Autodesk Inventor part; units mm, degrees
ref_plane "YZ Plane" through (0, 0, 0) normal (1, 0, 0) x (0, 1, 0)
ref_plane "XZ Plane" through (0, 0, 0) normal (0, 1, 0) x (-1, 0, 0)
ref_plane "XY Plane" through (0, 0, 0) normal (0, 0, 1) x (1, 0, 0)
sketch "Sketch1" plane through (0, 0, 0) normal (0, 1, 0) x (-1, 0, 0)
  circle A0 centre (0, 0) radius 2.0828
  dimension "d4" = 4.1656
extrude "Body" add sketch "Sketch1" along normal blind 6.35
sketch "Sketch2" plane through (0, 0, 0) normal (1, 0, 0) x (0, 1, 0)
  line L0 (6.35, -2.0828) -> (6.35, 2.0828)
  line L1 (6.35, 0) -> (6.35, -3.9624)
  line L2 (6.35, -3.9624) -> (6.731, -3.9624)
  arc A0 (6.731, -3.9624) -> (8.5598, -2.0828) centre (4.5388, 0) ccw
  line L3 (8.5598, -2.0828) -> (8.5598, -1.1938)
  line L4 (8.5598, -1.1938) -> (7.4676, -1.1938)
  line L5 (7.4676, -1.1938) -> (7.0866, -0.5588)
  line L6 (7.0866, -0.5588) -> (7.0866, 0)
  line L7 (7.0866, 0) -> (6.35, 0)
  point P0 (0, 0)
  dimension "d5" = 3.9624
  dimension "d6" = 0.381
  dimension "d13" = 0.7366
  dimension "d14" = 2.0828
  dimension "d15" = 2.2098
  dimension "d16" = 0
  dimension "d17" = 1.1938
  dimension "d18" = 0.5588
  dimension "d19" = 0.381
revolve "Head" add sketch "Sketch2" angle 360 about axis through (0, 7.0866, 0) along (0, -1, 0)
sketch "Sketch3" plane through (0, 8.5598, 0) normal (0, 1, 0) x (1, 0, 0)
  line L0 (0.6892, 1.1938) -> (1.3785, 0)
  line L1 (1.3785, 0) -> (0.6892, -1.1938)
  line L2 (0.6892, -1.1938) -> (-0.6892, -1.1938)
  line L3 (-0.6892, -1.1938) -> (-1.3785, 0)
  line L4 (-1.3785, 0) -> (-0.6892, 1.1938)
  line L5 (-0.6892, 1.1938) -> (0.6892, 1.1938)
  circle A0 centre (0, 0) radius 1.1938
  point P0 (0, 0)
  point P1 (0, 0)
extrude "Hex" cut sketch "Sketch3" against normal blind 1.1176
sketch "Sketch4" plane through (0, 0, 0) normal (0, 0, 1) x (1, 0, 0)
  line L0 (-0.6892, 7.4422) -> (0.6892, 7.4422)
  line L1 (-0.6892, 8.5598) -> (0.6892, 8.5598)
  line L2 (-0.254, 7.4422) -> (-1.3716, 8.5598)
  line L3 (-1.3785, 8.5598) -> (-1.3785, 7.4422)
  line L4 (-1.3785, 8.5598) -> (-0.254, 8.5598)
  line L5 (-0.254, 8.5598) -> (-0.254, 7.4422)
  line L6 (0, -4.252) -> (0, 25.5118)
  point P0 (0, 0)
  point P1 (0, 8.5598)
  point P2 (-0.254, 8.5598)
  dimension "d28" = 45
  dimension "d29" = 1.3716
revolve "Head Chamfer" cut sketch "Sketch4" angle 360 about axis through (0, -10, 0) along (0, 1, 0) contours L2 L4 L1 L5
sketch "Sketch5" plane through (0, 0, 0) normal (1, 0, 0) x (0, 1, 0)
  line L0 (0, -2.0828) -> (6.35, -2.0828)
  line L1 (6.35, 3.9624) -> (6.35, -3.9624)
  line L2 (6.35, -2.0828) -> (6.35, 2.0828)
  line L3 (0.0745, -2.0828) -> (-0.2261, -2.6035)
  line L4 (-0.2261, -2.6035) -> (-0.3253, -2.6035)
  line L5 (-0.3253, -2.6035) -> (-0.626, -2.0828)
  line L6 (0.0686, -2.6035) -> (-0.7252, -2.6035) construction
  line L7 (-0.626, -2.0828) -> (0.0745, -2.0828)
  line L8 (0, -2.0828) -> (6.35, -2.0828)
  point P0 (0, 0)
  dimension "d31" = 30
  dimension "d32" = 60
  dimension "a" = 0.0992
  dimension "d46" = 0.7937
  dimension "d54" = 0.0686
  dimension "d55" = 0.5207
  dimension "d56" = 0.0992
feature "Thread" [suppressed]
sketch "Sketch6" plane through (0, 0, 0) normal (0, 0, 1) x (1, 0, 0)
  line L0 (0, 0) -> (-1.4859, 0)
  line L1 (2.0828, 0) -> (-2.0828, 0)
  line L2 (-1.4859, 0) -> (-2.4948, 1.0089)
  line L3 (-2.4948, 1.0089) -> (-2.9651, -1.2188)
  line L4 (-2.9651, -1.2188) -> (-1.4859, -1.2188)
  line L5 (-2.0828, 0) -> (-2.0828, 6.35)
  line L6 (-1.4859, -1.2188) -> (-1.4859, 0)
  line L7 (0, -5.1871) -> (0, 22.5907)
  point P0 (-2.0828, 0.5969)
  dimension "d49" = 1.4859
  dimension "d50" = 135
revolve "Tapered End" cut sketch "Sketch6" angle 360 about axis through (0, -10, 0) along (0, 1, 0)
equation "\"d56\" = a"
properties part number "Screw 8-32 Steel 2.500" material "VEX Steel"
Part model, mm, in its own coordinate system. A direction names the side the tool comes from. Coordinates: 2 decimals unless noted, no trailing zeros. Loops run counter-clockwise (first coordinate to the right, second up) from the corner with the lowest first, then second, coordinate; pieces in that order, holes last. Notation, with made-up numbers: (-17.5, 42.5) - (-1.5, 42.5) arc R23 ccw to (-1.5, 62.5) - close; hole circle Ø3 at (86, -12). An arc over 180 degrees is marked (long way). Write item = value, one per line. Start each with the question number.
Item 1: Wall check: L1, parallel to Y at x = 0, z = 0; L2, parallel to Z at x = -0.5, y = 5; L3, parallel to X at y = 1, z = -1. Give the ranges that are in metal, low to high. Write a range as from..to.
Item 2: Cut at A-A, the plane y = 4.25. Give the cut face in (x, z), and give its area (3 significant figures).
Item 3: Flat gauge pins, fed straight in: pin 1 Ø2 at (x, y) = (3, 7.5) entering from +Z; pin 2 Ø1.2 at (x, z) = (0.5, -0.5) entering from +Y; pin 3 Ø4 at (x, y) = (3, 6) entering from -Z. Where does each tip first touch, or does it go through?
Item 4: 3-axis set-ups, long thin cutter, end or side, ignore diameter. For faces 1 (the flat face through (1.029, 8.009, -0.605)), 2 (the cylindrical face through (-1.987, 3.433, -0.626)): which of +Z, -Z, +X, -X, +Y, -Y reach the whole face in a straight line?
Item 5: Mould opens along X. For faces 3 (the flat face through (0, 8, 1.194)), 4 (the flat face through (0, 0, 0)), 5 (the cylindrical face through (-3.93, 6.54, 0.52)) say: released by +X, released by -X, zero draft, split by the parting line, or undercut.
The answers:
q1.L1 = 0..7.09
q1.L2 = -2.02..2.02
q1.L3 = -1.83..1.83
q2.outline = circle Ø4.17 at (0, 0)
q2.area = 13.6 mm2
q3.pin_1 = 3.19
q3.pin_2 = 8.5
q3.pin_3 = -3.83
q4.face_1 = +Y
q4.face_2 = -Y
q5.face_3 = undercut
q5.face_4 = zero draft
q5.face_5 = split by the parting line
